For this review, take the finished solid that the model builds, in its own axes (mm). A direction names the side the tool comes from. Coordinates: 2 decimals unless noted, no trailing zeros. Order: outer loops, then holes, each group sorted by start corner. A loop starts at its lowest first (then second) coordinate and runs counter-clockwise, first axis right, second up. Notation, with made-up numbers: (-13.5, -38) -> (32.5, -38) arc R23 ccw to (32.5, -30) -> close; hole circle Ø8 at (74.5, 16). An arc over 180 degrees is marked (long way). Return JSON: item names as keys, results as strings. Group by question number.
Item 1: Take a section at C-C (x = -4.5). Write out the cut boundary in (y, z), then the cut area to 4 significant figures.
Item 2: Take a section at A-A (y = 25.25). Write out the cut boundary in (x, z).
Item 3: Take a section at D-D (y = 15). Write out the cut boundary in (x, z), then the cut area to 3 significant figures.
Item 4: For line 1 along Y through (x, z) = (-4.5, 1.4); line 2 along X through (y, z) = (4, 0.55); line 3 along Y through (x, z) = (3, 0.4), list the stretches that pass through material, from the lowest coordinate up.
Item 5: Machinability: for faces 1 (the flat face through (0, 15, 1)), 2 (the flat face through (-9, 15, 1)), 3 (the flat face through (-5, 9, 3)), which of the approach directions +Z, -Z, +X, -X, +Y, -Y give a long, thin tool a straight path to every point of the face, cutting with its end or side? Answer none if there is none.
Item 6: Insertion check: pin 1 (0.9 mm diameter, centred on x = 2.5, z = 2, fed in from +Y). The pin has a flat end and moves straight along its axis. Give the tip position at first contact, or say it passes through.
```python
from build123d import *

# Parameters (mm, degrees)
ESQUISSE1_R        = 2.6
BOSS_EXTRU_1_DEPTH = 3
CONG_1_R           = 5
CONG_2_R           = 5


with BuildPart() as part:
    # Esquisse1 → Boss.-Extru.1 (new body)
    with BuildSketch(Plane.XY):
        Polygon((-9, 0), (-18, 0), (-18, -5), (9, -5), (9, 0), (0, 0), (0, 29.75), (-9, 29.75), align=None)
        with Locations((-4.5, 25.25)):
            Circle(ESQUISSE1_R, mode=Mode.SUBTRACT)
    extrude(amount=BOSS_EXTRU_1_DEPTH)

    # Congé1
    cong_1_edges = [part.edges().sort_by_distance(p)[0] for p in [
        (-18, 0, 1.5),
    ]]
    fillet(cong_1_edges, radius=CONG_1_R - 0.0001)  # a hair under: the kernel refuses the full size

    # Congé2
    cong_2_edges = [part.edges().sort_by_distance(p)[0] for p in [
        (9, 0, 1.5),
    ]]
    fillet(cong_2_edges, radius=CONG_2_R - 0.0001)  # a hair under: the kernel refuses the full size


solid = part.part
```
Findings below:
{
 "1": {"outline": "(-5, 0) -> (22.65, 0) -> (22.65, 3) -> (-5, 3) -> close; (27.85, 0) -> (29.75, 0) -> (29.75, 3) -> (27.85, 3) -> close", "area": "88.65 mm2"},
 "2": {"outline": "(-9, 0) -> (-7.1, 0) -> (-7.1, 3) -> (-9, 3) -> close; (-1.9, 0) -> (0, 0) -> (0, 3) -> (-1.9, 3) -> close"},
 "3": {"outline": "(-9, 0) -> (0, 0) -> (0, 3) -> (-9, 3) -> close", "area": "27.0 mm2"},
 "4": {"line 1": "y = -5 to 22.65, 27.85 to 29.75", "line 2": "x = -9 to 0", "line 3": "y = -5 to 0"},
 "5": {"face 1": "+Z, -Z, +X, +Y", "face 2": "+Z, -Z, -X, +Y", "face 3": "+Z, +X, -X, +Y, -Y"},
 "6": {"pin 1": "stops at y = 0"}
}
